Check sheet for the drawn part. Datum: minimum x, y, z corner. Units: mm. A direction names the side the tool comes from. Coordinates: 2 decimals unless noted, no trailing zeros. Write each loop counter-clockwise with the first axis right and the second up, starting at its lowest first coordinate (ties: lowest second). Pieces come first, ordered by that corner, then holes. Notation, with made-up numbers: (46, 82) -> (64, 82) arc R20 cw to (64, 105) -> close; hole circle Ø6 at (80, 66.5). An arc over 180 degrees is marked (long way). Answer in a Markdown table with one row per item.
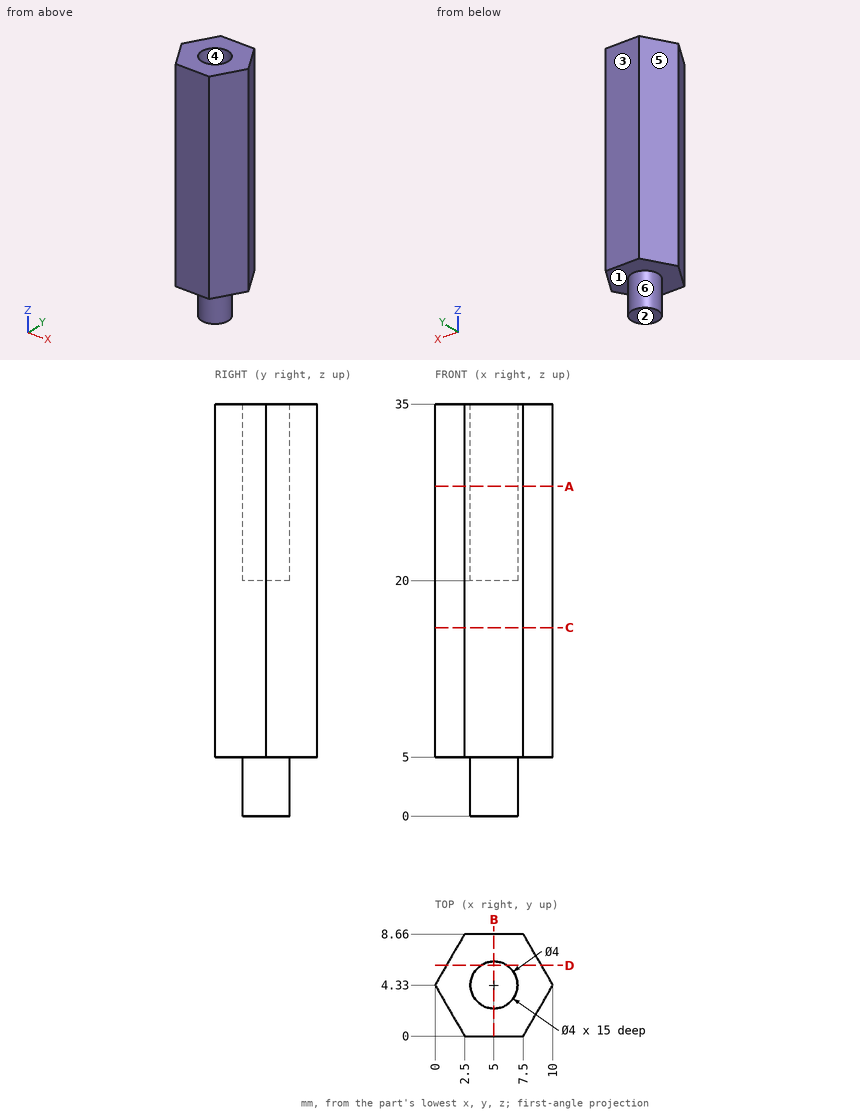
1. Material ranges on probe 1 along Z at (x, y) = (8, 7.5); probe 2 along X at (y, z) = (5.75, 29); probe 3 along Y at (x, z) = (5.5, 23.5), recorded low to high. Write a range as from..to.
Findings below:
| item | result |
|---|---|
| probe 1 | z = 5..35 |
| probe 2 | x = 0.82..3.59, 6.41..9.18 |
| probe 3 | y = 0..2.39, 6.27..8.66 |
2. Release check for a two-part mould opening along X. For the marked faces 3, 4, 5 and 6 record: released by +X, released by -X, zero draft, split by the parting line, or undercut.
Findings below:
| item | result |
|---|---|
| face 3 | zero draft |
| face 4 | undercut |
| face 5 | released by -X |
| face 6 | split by the parting line |
3. Go/stop test with flat-tipped pins: pin 1 (1.2 mm diameter, centred on x = 5, y = 5, fed in from +Z); pin 2 (4 mm diameter, centred on y = 7, z = 23, fed in from -X); pin 3 (1 mm diameter, centred on y = 2, z = 12.5, fed in from -X). Record where each tip stops, or that it passes through.
Findings below:
| item | result |
|---|---|
| pin 1 | stops at z = 20 |
| pin 2 | stops at x = 0.39 |
| pin 3 | stops at x = 1.06 |
4. Sectioned sample at C-C, the plane z = 16. Record the cut outline in (x, y).
Findings below:
| item | result |
|---|---|
| outline | (0, 4.33) -> (2.5, 0) -> (7.5, 0) -> (10, 4.33) -> (7.5, 8.66) -> (2.5, 8.66) -> close |
5. Sectioned sample at D-D, the plane y = 6. Record the cut outline in (x, z).
Findings below:
| item | result |
|---|---|
| outline | (0.96, 5) -> (3.9, 5) -> (3.9, 0) -> (6.1, 0) -> (6.1, 5) -> (9.04, 5) -> (9.04, 35) -> (6.1, 35) -> (6.1, 20) -> (3.9, 20) -> (3.9, 35) -> (0.96, 35) -> close |
6. Access from +Z, -Z, +X, -X, +Y, -Y to the whole of each face (thin tool, end or side, straight path). Record for the marked faces 1 and 2.
Findings below:
| item | result |
|---|---|
| face 1 | -Z |
| face 2 | -Z, +X, -X, +Y, -Y |
7. Sectioned sample at B-B, the plane x = 5. Record the cut outline in (y, z).
Findings below:
| item | result |
|---|---|
| outline | (0, 5) -> (2.33, 5) -> (2.33, 0) -> (6.33, 0) -> (6.33, 5) -> (8.66, 5) -> (8.66, 35) -> (6.33, 35) -> (6.33, 20) -> (2.33, 20) -> (2.33, 35) -> (0, 35) -> close |
8. Sectioned sample at A-A, the plane z = 28. Record the cut outline in (x, y).
Findings below:
| item | result |
|---|---|
| outline | (0, 4.33) -> (2.5, 0) -> (7.5, 0) -> (10, 4.33) -> (7.5, 8.66) -> (2.5, 8.66) -> close; hole circle Ø4 at (5, 4.33) |
